from build123d import *

# Parameters (mm, degrees)
BOSS_EXTRUDE1_DEPTH  = 100
M6_CLEARANCE_HOLE2_D = 6.6
CHAMFER1_SIZE        = 0.6


with BuildPart() as part:
    # Sketch1 → Boss-Extrude1 (new body)
    with BuildSketch(Plane.XY):
        Polygon((-61, 0), (-56, 0), (-56, 0.8), (-27.5, 0.8), (-27.5, 2.8), (-39.624355653, 9.8), (-61, 9.8), align=None)
    extrude(amount=BOSS_EXTRUDE1_DEPTH)

    # M6 Clearance Hole2 (through all)
    with Locations(Plane(origin=(0, 9.8, 0), x_dir=(1, 0, 0), z_dir=(0, 1, 0))):
        with Locations((-50, -92.5), (-50, -7.5)):
            Hole(M6_CLEARANCE_HOLE2_D / 2)

    # Chamfer1
    chamfer1_edges = [part.edges().sort_by_distance(p)[0] for p in [
        (-61, 9.8, 50),
        (-46.7, 9.8, 92.5),
        (-50.312177826, 9.8, 100),
        (-46.7, 9.8, 7.5),
        (-50.312177826, 9.8, 0),
    ]]
    chamfer(chamfer1_edges, length=CHAMFER1_SIZE)


solid = part.part
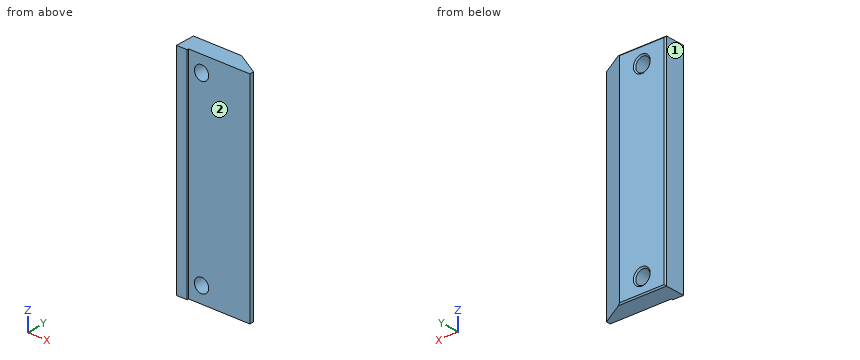
Verification items for the finished model (mm, model axes). Face numbers are marked on the shaded views. A direction names the side the tool comes from. Round coordinates to 2 decimals unless told otherwise and drop trailing zeros. Loops run counter-clockwise (first coordinate to the right, second up) from the corner with the lowest first, then second, coordinate; pieces in that order, holes last. Notation, with made-up numbers: (-14, -8) - (36, -8) arc R28 ccw to (36, 11) - close; hole circle Ø5 at (16.25, 43). An arc over 180 degrees is marked (long way). Answer in a Markdown table with one row per item. Add a question column.
Q1. Material ranges on line 1 (Z direction, x = -50, y = 2.5); line 2 (Z direction, x = -52.5, y = 7.75); line 3 (Y direction, x = -54.5, z = 14), recorded low to high.
Q2. Gauge pin test, flat ends, axial feed: pin 1 (10.5 mm diameter, centred on x = -50, z = 7.5, fed in from -Y); pin 2 (4 mm diameter, centred on x = -50, z = 92.5, fed in from -Y); pin 3 (2 mm diameter, centred on y = 6, z = 46.5, fed in from +X); pin 4 (5 mm diameter, centred on x = -32.5, z = 68, fed in from +Y). Record the tip position at first contact, or that the pin passes through.
Q3. Tool access check on the marked faces 1 and 2. Record the directions out of +Z, -Z, +X, -X, +Y, -Y that give a thin tool (end or side, any length) a straight path to the whole face; none if there is none.
Q4. Section check B-B on x = -42. Enter the section's corners in (y, z).
Q5. Section check C-C on z = 56. Enter the section's corners in (x, y), plus the area to 3 significant figures.
Q6. Section check A-A on z = 92.5. Enter the section's corners in (x, y), plus the area to 3 significant figures.
Q7. Section check D-D on x = -48.5. State how many separate pieces and enclosed holes the cut face has, plus the area to 3 significant figures.
Found:
| question | item | result |
|---|---|---|
| 1 | line 1 | z = 0 to 4.2, 10.8 to 89.2, 95.8 to 100 |
| 1 | line 2 | z = 0 to 5.35, 9.65 to 90.35, 94.65 to 100 |
| 1 | line 3 | y = 0.8 to 9.8 |
| 2 | pin 1 | stops at y = 0.8 |
| 2 | pin 2 | passes through |
| 2 | pin 3 | stops at x = -31.31 |
| 2 | pin 4 | stops at y = 7.13 |
| 3 | face 1 | +Z, -Z, -X, +Y, -Y |
| 3 | face 2 | +Z, -Z, +X, -Y |
| 4 | outline | (0.8, 0) - (9.2, 0) - (9.8, 0.6) - (9.8, 99.4) - (9.2, 100) - (0.8, 100) - close |
| 5 | outline | (-61, 0) - (-56, 0) - (-56, 0.8) - (-27.5, 0.8) - (-27.5, 2.8) - (-39.62, 9.8) - (-60.4, 9.8) - (-61, 9.2) - close |
| 5 | area | 263 mm² |
| 6 | outline | (-61, 0) - (-56, 0) - (-56, 0.8) - (-53.3, 0.8) - (-53.3, 9.2) - (-53.9, 9.8) - (-60.4, 9.8) - (-61, 9.2) - close; (-46.7, 0.8) - (-27.5, 0.8) - (-27.5, 2.8) - (-39.62, 9.8) - (-46.1, 9.8) - (-46.7, 9.2) - close |
| 6 | area | 203 mm² |
| 7 | separate pieces | 3 |
| 7 | enclosed holes | 0 |
| 7 | area | 793 mm² |
